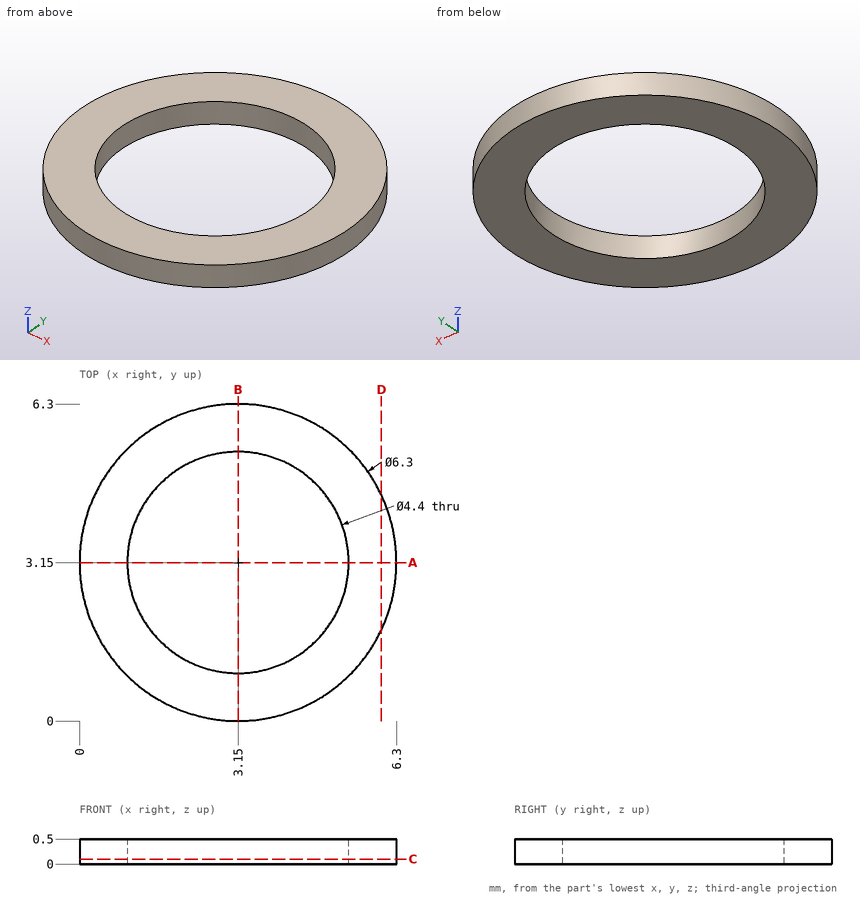
Check sheet for the drawn part. Datum: minimum x, y, z corner. Units: mm. Coordinates: 2 decimals unless noted, no trailing zeros. Order: outer loops, then holes, each group sorted by start corner. A loop starts at its lowest first (then second) coordinate and runs counter-clockwise, first axis right, second up. Notation, with made-up numbers: M 82,-10.75 L 126,-10.75 A25 ccw 126,22.25 Z; hole C 87.25,-30.5 d9. An arc over 180 degrees is marked long. One line per question, with ' | ' between items. Start each with the question number.
Item 1: Sectioned sample at A-A on y = 3.15. Record the cut outline in (x, z).
Item 2: Sectioned sample at C-C on z = 0.1. Record the cut outline in (x, y).
Item 3: Material ranges on line 1 (Y direction, x = 3.15, z = 0.35); line 2 (Y direction, x = 1.75, z = 0.1), recorded low to high.
Item 4: Sectioned sample at D-D on x = 6. Record the cut outline in (y, z).
Answer below:
1) outline: M 0,0 L 0.95,0 L 0.95,0.5 L 0,0.5 Z; M 5.35,0 L 6.3,0 L 6.3,0.5 L 5.35,0.5 Z
2) outline: C 3.15,3.15 d6.3; hole C 3.15,3.15 d4.4
3) line 1: y = 0 to 0.95, 5.35 to 6.3 | line 2: y = 0.33 to 1.45, 4.85 to 5.97
4) outline: M 1.81,0 L 4.49,0 L 4.49,0.5 L 1.81,0.5 Z
